Here's the drawing with two shaded views (mm, measured from the low corner). I have some questions. Coordinates: 2 decimals unless noted, no trailing zeros. Write each loop counter-clockwise with the first axis right and the second up, starting at its lowest first coordinate (ties: lowest second). Pieces come first, ordered by that corner, then holes.
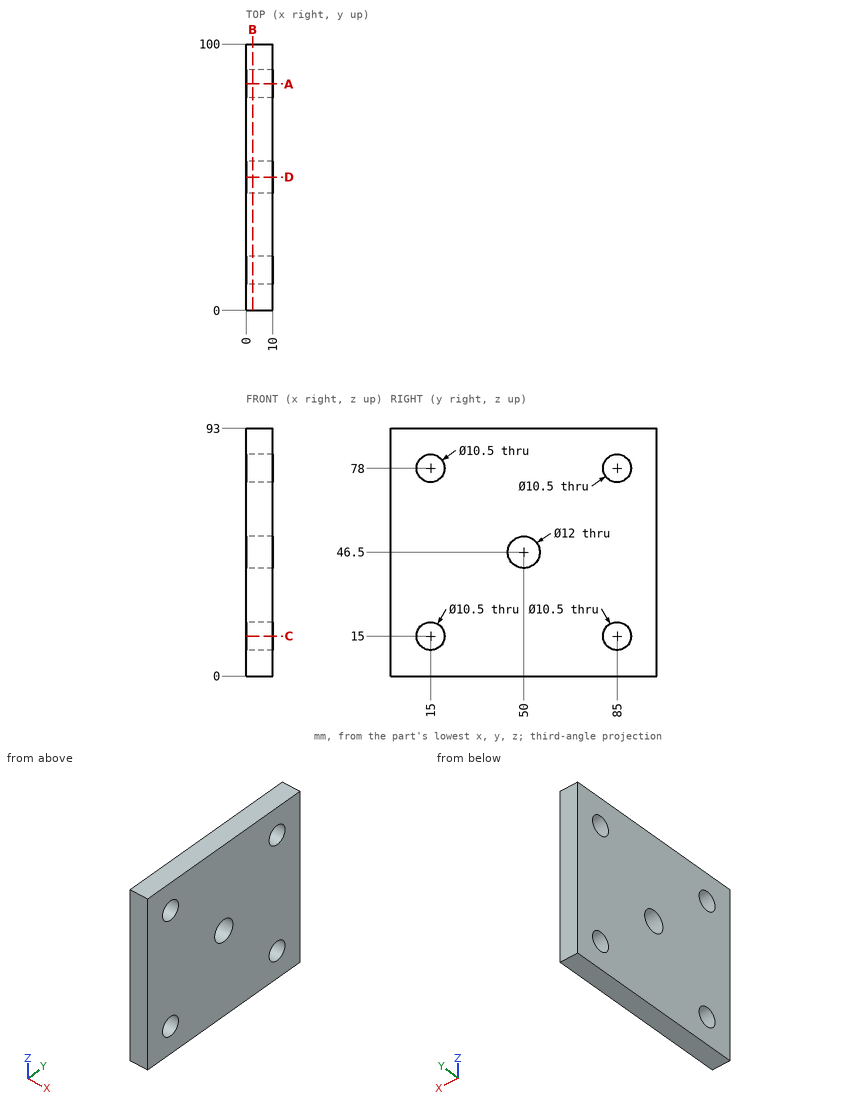
Item 1: I want a section at B-B, the plane x = 2.5. List the corners of the cut face in (y, z) for me.
Item 2: I want a section at A-A, the plane y = 85. List the corners of the cut face in (x, z) for me.
Item 3: I want a section at C-C, the plane z = 15. List the corners of the cut face in (x, y) for me, then the cut area to 3 significant figures.
Item 4: If I drill on line 1 along Z through (x, y) = (6.5, 15); line 2 along Z through (x, y) = (8.75, 50); line 3 along Z through (x, y) = (1.5, 13.5), over which ranges is the centre line in solid material (lowest first)?
Item 5: Will this pin go through, and if not, where does the flat tip stop? pin 1 Ø8.5 at (y, z) = (85, 78) entering from +X.
Item 6: I want a section at D-D, the plane y = 50. List the corners of the cut face in (x, z) for me, then the cut area to 3 significant figures.
Taken from the geometry:
1. outline: (0, 0) - (100, 0) - (100, 93) - (0, 93) - close; hole circle Ø10.5 at (15, 15); hole circle Ø10.5 at (15, 78); hole circle Ø12 at (50, 46.5); hole circle Ø10.5 at (85, 15); hole circle Ø10.5 at (85, 78)
2. outline: (0, 0) - (10, 0) - (10, 9.75) - (0, 9.75) - close; (0, 20.25) - (10, 20.25) - (10, 72.75) - (0, 72.75) - close; (0, 83.25) - (10, 83.25) - (10, 93) - (0, 93) - close
3. outline: (0, 0) - (10, 0) - (10, 9.75) - (0, 9.75) - close; (0, 20.25) - (10, 20.25) - (10, 79.75) - (0, 79.75) - close; (0, 90.25) - (10, 90.25) - (10, 100) - (0, 100) - close
3. area: 790 mm2
4. line 1: z = 0 to 9.75, 20.25 to 72.75, 83.25 to 93
4. line 2: z = 0 to 40.5, 52.5 to 93
4. line 3: z = 0 to 9.97, 20.03 to 72.97, 83.03 to 93
5. pin 1: passes through
6. outline: (0, 0) - (10, 0) - (10, 40.5) - (0, 40.5) - close; (0, 52.5) - (10, 52.5) - (10, 93) - (0, 93) - close
6. area: 810 mm2
